Can you work these out from the model? Positions are in its coordinate system, mm. A direction names the side the tool comes from. Round coordinates to 2 decimals unless told otherwise and drop trailing zeros. Loops run counter-clockwise (first coordinate to the right, second up) from the corner with the lowest first, then second, coordinate; pieces in that order, holes last. Notation, with made-up numbers: (-14.75, 7) -> (42.25, 7) arc R18 cw to (42.25, 30) -> close; hole circle Ø9 at (-33.5, 47). An arc over 180 degrees is marked (long way). Write each question's results on one line, items separated by ' | '.
from build123d import *

# Parameters (mm, degrees)
F0_R     = 13
F1_DEPTH = 38
F0_R_2   = 10
F2_DEPTH = 19


with BuildPart() as f1:
    # F0 (on Top) → F1 (new body)
    with BuildSketch(Plane.XY):
        with BuildLine():
            ThreePointArc((18.895579, -21.999025), (26.3531, -12.104301), (29, 0))
            ThreePointArc((29, 0), (26.353016, 12.104485), (18.895272, 21.999288))
            ThreePointArc((18.895272, 21.999288), (0.000503, 29), (-18.894509, 21.999944))
            ThreePointArc((-18.894509, 21.999944), (-29, -3.2e-05), (-18.894461, -21.999985))
            ThreePointArc((-18.894461, -21.999985), (0.000737, -29), (18.895579, -21.999025))
        make_face()
        Circle(F0_R, mode=Mode.SUBTRACT)
    extrude(amount=F1_DEPTH)

    # F0 (on Top) → F2 (join)
    with BuildSketch(Plane.XY):
        with BuildLine():
            ThreePointArc((18.895272, 21.999288), (26.353016, 12.104485), (29, 0))
            ThreePointArc((29, 0), (26.3531, -12.104301), (18.895579, -21.999025))
            Line((18.895579, -21.999025), (47.792855, -21.999025))
            Line((47.792855, -21.999025), (48.207145, -21.999025))
            ThreePointArc((48.207145, -21.999025), (69.999162, 0.192041), (47.823064, 21.999288))
            Line((47.823064, 21.999288), (18.895272, 21.999288))
        make_face()
        with Locations((48, 0)):
            Circle(F0_R_2, mode=Mode.SUBTRACT)
        with BuildLine():
            ThreePointArc((-18.894461, -21.999985), (-29, -3.2e-05), (-18.894509, 21.999944))
            Line((-18.894509, 21.999944), (-47.950196, 21.999944))
            ThreePointArc((-47.950196, 21.999944), (-48, 22), (-48.049804, 21.999944))
            ThreePointArc((-48.049804, 21.999944), (-69.999997, -0.012047), (-48.025711, -21.999985))
            ThreePointArc((-48.025711, -21.999985), (-48, -22), (-47.974289, -21.999985))
            Line((-47.974289, -21.999985), (-18.894461, -21.999985))
        make_face()
        with Locations((-48, 0)):
            Circle(F0_R_2, mode=Mode.SUBTRACT)
    extrude(amount=F2_DEPTH)


solid = f1.part
1. Please list where these lines run through material, in increasing order: line 1 (Y direction, x = 0, z = 22); line 2 (Y direction, x = -48, z = 6); line 3 (X direction, y = 1, z = 5). Write a range as from..to.
Final values:
line 1: -29..-13, 13..29 | line 2: -22..-10, 10..22 | line 3: -69.98..-57.95, -38.05..-12.96, 12.96..38.05, 57.95..69.98
2. If we section it at C-C (y = -8): List the corners of the cut face in (x, z) for me, then the cut area to 3 significant figures.
Final values:
outline: (-68.49, 0) -> (-54, 0) -> (-54, 19) -> (-68.49, 19) -> close; (-42, 0) -> (-10.25, 0) -> (-10.25, 38) -> (-27.87, 38) -> (-27.87, 19) -> (-42, 19) -> close; (10.25, 0) -> (42, 0) -> (42, 19) -> (27.87, 19) -> (27.87, 38) -> (10.25, 38) -> close; (54, 0) -> (68.49, 0) -> (68.49, 19) -> (54, 19) -> close | area: 2,430 mm2
3. Will these pins go through, and if not, where does the flat tip stop? pin 1 (9.5 mm diameter, centred on x = 31.5, z = 13.5, fed in from +Y); pin 2 (3 mm diameter, centred on x = -34.5, y = -23, fed in from +Z); pin 3 (13 mm diameter, centred on x = -48, y = -1.5, fed in from +Z) (1 decimal); pin 4 (5.5 mm diameter, centred on x = -40.5, z = 7, fed in from -Y).
Final values:
pin 1: y = 22 | pin 2: z = 19 | pin 3: through | pin 4: y = -22
4. If we section it at B-B (z = 21): List the corners of the cut face in (x, y) for me, then the cut area to 3 significant figures.
Final values:
outline: (18.9, -22) arc R29 ccw to (29, 0) arc R29 ccw to (18.9, 22) arc R29 ccw (long way) to start; hole circle Ø26 at (0, 0) | area: 2,110 mm2
5. On a 3-axis mill with a long thin cutter (end or side, diameter ignored), from which of +Z, -Z, +X, -X, +Y, -Y can I reach the whole of each face in a straight line? I mean faces 1 (the face through (-10.316, -7.91, 18.734)), 2 (the face through (34, 21.999, 9)), 3 (the face through (-34, -22, 9)), 4 (the face through (-33, 22, 9)), 5 (the face through (33, -21.999, 9)). Say none if no direction works.
Final values:
face 1: +Z, -Z | face 2: +Z, -Z, +X, +Y | face 3: +Z, -Z, -X, -Y | face 4: +Z, -Z, -X, +Y | face 5: +Z, -Z, +X, -Y
6. If we section it at A-A (x = 0): List the corners of the cut face in (y, z) for me.
Final values:
outline: (-29, 0) -> (-13, 0) -> (-13, 38) -> (-29, 38) -> close; (13, 0) -> (29, 0) -> (29, 38) -> (13, 38) -> close
7. If we section it at D-D (y = 18.5): List the corners of the cut face in (x, z) for me.
Final values:
outline: (-59.91, 0) -> (59.91, 0) -> (59.91, 19) -> (22.33, 19) -> (22.33, 38) -> (-22.33, 38) -> (-22.33, 19) -> (-59.91, 19) -> close
8. We'd pull the mould along X, two halves only. Please class faces 6 (the face through (-70, 0, 9)), 7 (the face through (12, -6, 38)), 8 (the face through (-58, 0, 9)): pulls with the +X half, pulls with the -X half, needs draft (parallel to the pull), parting line crosses it, or undercut.
Final values:
face 6: pulls with the -X half | face 7: needs draft | face 8: undercut
